Study the drawing (mm; zero at the part's minimum x, y, z) and answer. A direction names the side the tool comes from. Coordinates: 2 decimals unless noted, no trailing zeros. Order: outer loops, then holes, each group sorted by start corner. A loop starts at its lowest first (then second) coordinate and runs counter-clockwise, first axis right, second up. Notation, with made-up numbers: (4.25, 67.25) -> (49.25, 67.25) arc R15 ccw to (49.25, 83.25) -> close; hole circle Ø8 at (-0.75, 24.25). An arc over 180 degrees is marked (long way). Write each question's results on one line, items separated by ' | '. Start each with the question number.
(1) Given pin 1 (6 mm diameter, centred on x = 17, y = 6.5, fed in from +Z), flat-ended and moving along its own axis, determine where the tip first touches the part or whether it passes through.
(2) A straight line is drawn through the part: L1, parallel to Y at x = 10, z = 78. Find the intervals that lie inside material, in ascending order.
(3) A tool of negligible diameter and unlimited length cuts with its end or side. For the marked faces 5 and 6, from which of +Z, -Z, +X, -X, +Y, -Y can it reach the whole face along a straight path? Write none if from no direction.
(4) The part is cut by section A-A, the plane z = 151. Give the vertices of the cut face in (x, y), then the cut area to 3 significant figures.
(5) The part is cut by section B-B, the plane x = 8.75. Give the vertices of the cut face in (y, z).
(6) Determine the mould class of the marked faces 1, 2, 3 and 4 for opening direction X: +X half, -X half, draft (parallel to the pull), parting line (faces both ways), or undercut.
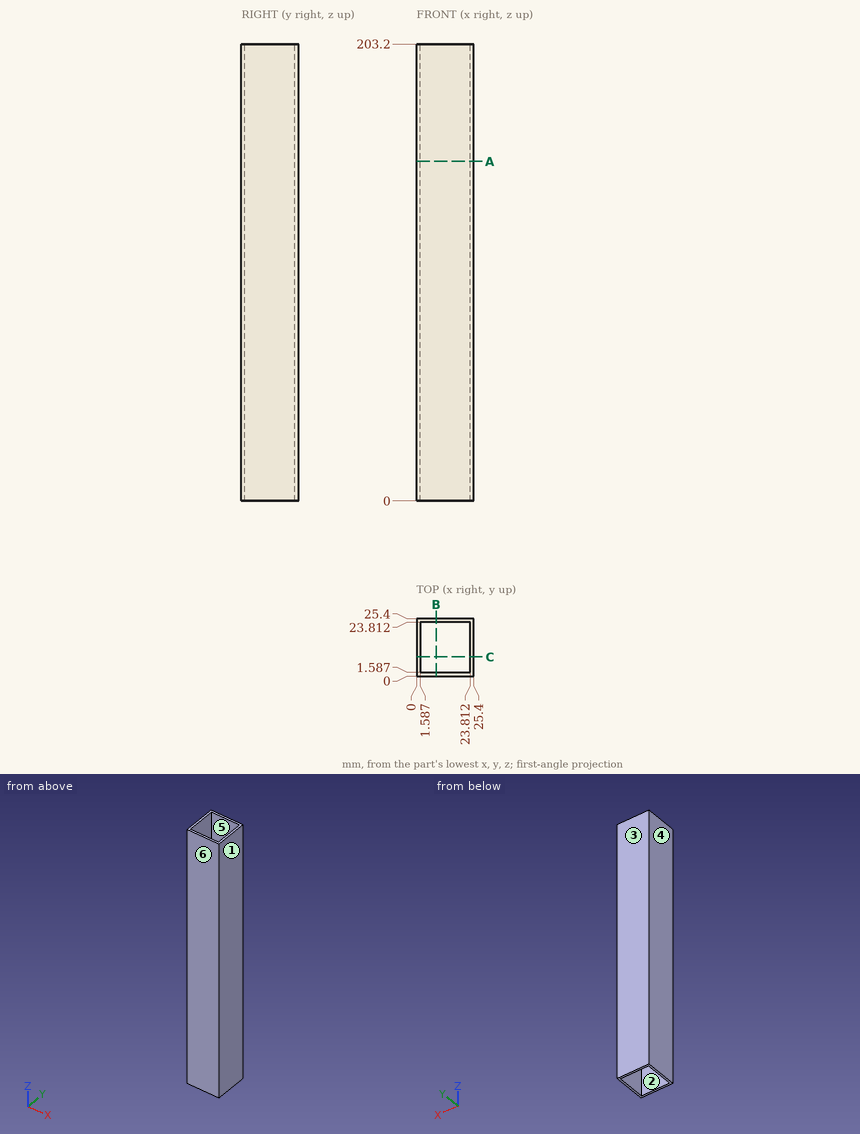
Established:
1) pin 1: passes through
2) L1: y = 0 to 1.59, 23.81 to 25.4
3) face 5: +Z, -Z | face 6: +Z, -Z, +X, -X, -Y
4) outline: (0, 0) -> (25.4, 0) -> (25.4, 25.4) -> (0, 25.4) -> close; hole (1.59, 1.59) -> (23.81, 1.59) -> (23.81, 23.81) -> (1.59, 23.81) -> close | area: 151 mm^2
5) outline: (0, 0) -> (1.59, 0) -> (1.59, 203.2) -> (0, 203.2) -> close; (23.81, 0) -> (25.4, 0) -> (25.4, 203.2) -> (23.81, 203.2) -> close
6) face 1: +X half | face 2: undercut | face 3: draft | face 4: -X half
